The model under review builds one solid part; all positions refer to its coordinate system, in mm. Face numbers are marked on the shaded views. A direction names the side the tool comes from. Round coordinates to 2 decimals unless told otherwise and drop trailing zeros. Order: outer loops, then holes, each group sorted by start corner. A loop starts at its lowest first (then second) coordinate and runs counter-clockwise, first axis right, second up. Notation, with made-up numbers: M 53,-37.75 L 86,-37.75 A13 ccw 86,-20.75 Z; hole C 85.25,30.5 d2. An arc over 180 degrees is marked long. Answer as a JSON object with one key per item and string values. Group by question number.
1. To check wall thickness, follow probe 1 along X at (y, z) = (-17, 0); probe 2 along Y at (x, z) = (39.5, 17); probe 3 along Y at (x, z) = (-4, -52). State the ranges of each line that lie inside material, in increasing order. Write a range as [from, to].
2. Add section D-D on x = 0. State the section outline as (y, z) points, and give its area (3 significant figures).
3. Add section A-A on y = 18. State the section outline as (x, z) points, and give its area (3 significant figures).
4. Machinability: for the marked faces 1, 2 and 3, which of the approach directions +Z, -Z, +X, -X, +Y, -Y give a long, thin tool a straight path to every point of the face, cutting with its end or side? Answer none if there is none.
5. Mouldability with a two-part tool opening along X and no side actions: class the marked faces 4, 5 and 6 as released by +X, released by -X, zero draft, split by the parting line, or undercut.
6. Add section B-B on z = 0. State the section outline as (x, y) points.
7. Clearance check with flat-ended pins moving along their axes: P1, Ø1.5, axis at y = -10.5, z = 15.5, coming from the -X side; P2, Ø5, axis at x = 1.5, y = -18.5, coming from the -Z side; P3, Ø4, axis at y = -12, z = 16.5, coming from the +X side; P4, Ø1, axis at x = 37.5, y = -2, coming from the +Z side. State where each tip first meets the part, or that it passes through.
8. Add section C-C on y = -19.5. State the section outline as (x, z) points, and give its area (3 significant figures).
```python
from build123d import *

# Parameters (mm, degrees)
SKETCH2_R           = 60
BOSS_EXTRUDE1_DEPTH = 25
SKETCH3_R           = 30
BOSS_EXTRUDE2_DEPTH = 30
SKETCH4_R           = 15
CUT_EXTRUDE1_DEPTH  = 30
SKETCH5_W           = 10
SKETCH5_H           = 8
CUT_EXTRUDE2_DEPTH  = 30
SKETCH6_W           = 15
SKETCH6_H           = 130
CUT_EXTRUDE3_DEPTH  = 15
FILLET1_R           = 2
FILLET2_R           = 1.5


with BuildPart() as part:
    # Sketch2 → Boss-Extrude1 (new body)
    with BuildSketch(Plane(origin=(0, 0, 0), x_dir=(-1, 0, 0), z_dir=(0, 1, 0))):
        with Locations(Location((0, 0, 0), (0, 0, 90))):
            Circle(SKETCH2_R)
    extrude(amount=BOSS_EXTRUDE1_DEPTH)

    # Sketch3 → Boss-Extrude2 (add)
    with BuildSketch(Plane.XZ):
        with Locations(Location((0, 0, 0), (0, 0, 270))):
            Circle(SKETCH3_R)
    extrude(amount=BOSS_EXTRUDE2_DEPTH)

    # Sketch4 → Cut-Extrude1 (cut)
    with BuildSketch(Plane.XZ.offset(30)):
        with Locations(Location((0, 0, 0), (0, 0, 270))):
            Circle(SKETCH4_R)
    extrude(amount=-CUT_EXTRUDE1_DEPTH, mode=Mode.SUBTRACT)

    # Sketch5 → Cut-Extrude2 (cut)
    with BuildSketch(Plane.XZ.offset(30)):
        with Locations((0, 15)):
            Rectangle(SKETCH5_W, SKETCH5_H)
    extrude(amount=-CUT_EXTRUDE2_DEPTH, mode=Mode.SUBTRACT)

    # Sketch6 → Cut-Extrude3 (cut)
    with BuildSketch(Plane(origin=(0, 25, 0), x_dir=(-1, 0, 0), z_dir=(0, 1, 0))):
        Rectangle(SKETCH6_W, SKETCH6_H)
    extrude(amount=-CUT_EXTRUDE3_DEPTH, mode=Mode.SUBTRACT)

    # Fillet1
    fillet1_edges = [part.edges().sort_by_distance(p)[0] for p in [
        (0, 0, -60),
    ]]
    fillet(fillet1_edges, radius=FILLET1_R)

    # Fillet2
    fillet2_edges = [part.edges().sort_by_distance(p)[0] for p in [
        (-60, 25, 0),
        (7.5, 25, 0),
        (-7.5, 25, 0),
        (0, 10, -60),
        (3.757374753, 10, 59.882235554),
        (-7.5, 17.5, -59.529404499),
        (-7.5, 10, 0),
        (-7.5, 17.5, 59.529404499),
        (7.5, 17.5, 59.529404499),
        (7.5, 10, 0),
        (7.5, 17.5, -59.529404499),
        (60, 25, 0),
    ]]
    fillet(fillet2_edges, radius=FILLET2_R)


solid = part.part
```
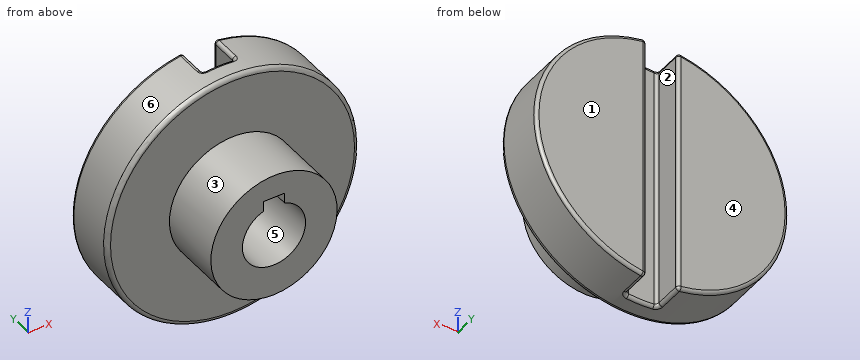
Recorded:
{
 "1": {"probe 1": "x = [-30, -15], [15, 30]", "probe 2": "y = [0, 25]", "probe 3": "y = [0, 10]"},
 "2": {"outline": "M -30,-30 L 0,-30 L 0,-58 A2 ccw 2,-60 L 8.5,-60 A1.5 ccw 10,-58.5 L 10,58.5 A1.5 ccw 8.5,60 L 2,60 A2 ccw 0,58 L 0,30 L -30,30 L -30,19 L 0,19 L 0,-15 L -30,-15 Z", "area": "1,980 mm²"},
 "3": {"outline": "M -9.23,-59.29 A1.5 ccw -7.5,-57.8 L -7.5,57.8 A1.5 ccw -9.23,59.29 A60 ccw Z; M 7.5,-57.8 A1.5 ccw 9.23,-59.29 A60 ccw 9.23,59.29 A1.5 ccw 7.5,57.8 Z", "area": "9,510 mm²"},
 "4": {"face 1": "+Z, -Z, +X, -X, +Y", "face 2": "+Z, -Z, +Y", "face 3": "-Y"},
 "5": {"face 4": "zero draft", "face 5": "undercut", "face 6": "split by the parting line"},
 "6": {"outline": "M -60,2 A2 ccw -58,0 L -30,0 L -30,-30 L -15,-30 L -15,0 L 15,0 L 15,-30 L 30,-30 L 30,0 L 58,0 A2 ccw 60,2 L 60,23.5 A1.5 ccw 58.5,25 L 9,25 A1.5 ccw 7.5,23.5 L 7.5,11.5 A1.5 cw 6,10 L -6,10 A1.5 cw -7.5,11.5 L -7.5,23.5 A1.5 ccw -9,25 L -58.5,25 A1.5 ccw -60,23.5 Z"},
 "7": {"P1": "stops at x = -26.12", "P2": "stops at z = -30", "P3": "stops at x = 26.26", "P4": "passes through"},
 "8": {"outline": "C 0,0 d60; hole M -5,14.14 A15 ccw long 5,14.14 L 5,19 L -5,19 Z", "area": "2,080 mm²"}
}
